Can you work these out from the model? Positions are in its coordinate system, mm. Face numbers are marked on the shaded views. A direction names the side the tool comes from. Coordinates: 2 decimals unless noted, no trailing zeros. Order: outer loops, then holes, each group sorted by start corner. A loop starts at its lowest first (then second) coordinate and runs counter-clockwise, first axis right, second up. Notation, with made-up numbers: (23.25, 83) -> (48.25, 83) arc R12 cw to (48.25, 94) -> close; hole circle Ø5 at (-6, 81.5). An arc over 180 degrees is marked (long way). Write item = value, one per line.
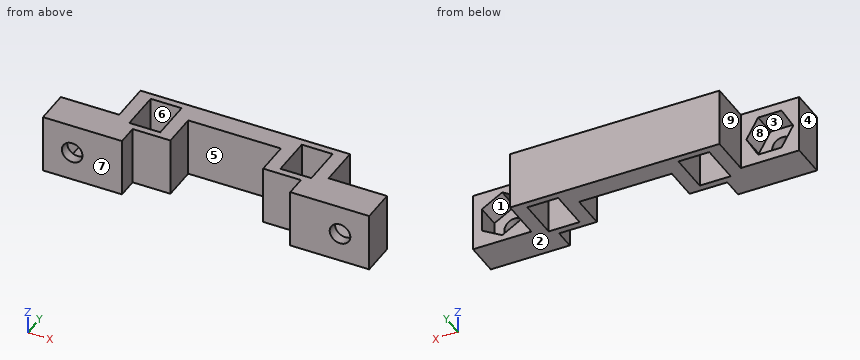
```python
from build123d import *

# Parameters (mm, degrees)
SKETCH1_W           = 8.5
SKETCH1_H           = 8.5
BOSS_EXTRUDE1_DEPTH = 3.5
SKETCH2_W           = 8.5
SKETCH2_H           = 8.5
SKETCH2_R           = 1.5
BOSS_EXTRUDE2_DEPTH = 1.5
SKETCH3_W           = 8.5
SKETCH3_H           = 5
BOSS_EXTRUDE3_DEPTH = 3
SKETCH4_W           = 3
SKETCH4_H           = 8.5
BOSS_EXTRUDE4_DEPTH = 6
SKETCH5_W           = 8.5
SKETCH5_H           = 3
BOSS_EXTRUDE5_DEPTH = 27.5
SKETCH6_W           = 3
SKETCH6_H           = 8.5
BOSS_EXTRUDE6_DEPTH = 8
SKETCH7_W           = 8.5
SKETCH7_H           = 5
BOSS_EXTRUDE7_DEPTH = 8.5
CUT_EXTRUDE1_DEPTH  = 3.5
SKETCH10_R          = 1.5
CUT_EXTRUDE3_DEPTH  = 3.5
BOSS_EXTRUDE8_REACH = 38
SKETCH15_W          = 8.5
SKETCH15_H          = 5
SKETCH16_W          = 4.5
SKETCH16_H          = 6
CUT_EXTRUDE4_DEPTH  = 10
SKETCH17_W          = 13.5
SKETCH17_H          = 5
CUT_EXTRUDE5_DEPTH  = 10


with BuildPart() as part:
    # Sketch1 → Boss-Extrude1 (new body)
    with BuildSketch(Plane(origin=(0, 0, 0), x_dir=(1, 0, 0), z_dir=(0, 1, 0))):
        with Locations((4.25, 4.25)):
            Rectangle(SKETCH1_W, SKETCH1_H)
        Polygon((5.985496764, 7.195964334), (2.575496764, 7.195964334), (0.870496764, 4.242817707), (2.575496764, 1.28967108), (5.985496764, 1.28967108), (7.690496764, 4.242817707), align=None, mode=Mode.SUBTRACT)
    extrude(amount=BOSS_EXTRUDE1_DEPTH)

    # Sketch2 → Boss-Extrude2 (add)
    with BuildSketch(Plane.XZ):
        with Locations((4.25, -4.25)):
            Rectangle(SKETCH2_W, SKETCH2_H)
        with Locations((4.25, -4.25)):
            Circle(SKETCH2_R, mode=Mode.SUBTRACT)
    extrude(amount=BOSS_EXTRUDE2_DEPTH)

    # Sketch3 → Boss-Extrude3 (add)
    with BuildSketch(Plane(origin=(8.5, 0, 0), x_dir=(0, 0, -1), z_dir=(1, 0, 0))):
        with Locations((4.25, 1)):
            Rectangle(SKETCH3_W, SKETCH3_H)
    extrude(amount=BOSS_EXTRUDE3_DEPTH)

    # Sketch4 → Boss-Extrude4 (add)
    with BuildSketch(Plane(origin=(0, 3.5, 0), x_dir=(1, 0, 0), z_dir=(0, 1, 0))):
        with Locations((10, 4.25)):
            Rectangle(SKETCH4_W, SKETCH4_H)
    extrude(amount=BOSS_EXTRUDE4_DEPTH)

    # Sketch5 → Boss-Extrude5 (add)
    with BuildSketch(Plane(origin=(11.5, 0, 0), x_dir=(0, 0, -1), z_dir=(1, 0, 0))):
        with Locations((4.25, 8)):
            Rectangle(SKETCH5_W, SKETCH5_H)
    extrude(amount=BOSS_EXTRUDE5_DEPTH)

    # Sketch6 → Boss-Extrude6 (add)
    with BuildSketch(Plane.XZ.offset(-6.5)):
        with Locations((37.5, -4.25)):
            Rectangle(SKETCH6_W, SKETCH6_H)
    extrude(amount=BOSS_EXTRUDE6_DEPTH)

    # Sketch7 → Boss-Extrude7 (add)
    with BuildSketch(Plane(origin=(39, 0, 0), x_dir=(0, 0, -1), z_dir=(1, 0, 0))):
        with Locations((4.25, 1)):
            Rectangle(SKETCH7_W, SKETCH7_H)
    extrude(amount=BOSS_EXTRUDE7_DEPTH)

    # Sketch8 → Cut-Extrude1 (cut)
    with BuildSketch(Plane(origin=(0, 3.5, 0), x_dir=(1, 0, 0), z_dir=(0, 1, 0))):
        Polygon((46.203146627, 5.955), (43.25, 7.66), (40.296853373, 5.955), (40.296853373, 2.545), (43.25, 0.84), (46.203146627, 2.545), align=None)
    extrude(amount=-CUT_EXTRUDE1_DEPTH, mode=Mode.SUBTRACT)

    # Sketch10 → Cut-Extrude3 (cut)
    with BuildSketch(Plane(origin=(0, 0, 0), x_dir=(1, 0, 0), z_dir=(0, 1, 0))):
        with Locations((43.25, 4.25)):
            Circle(SKETCH10_R)
    extrude(amount=-CUT_EXTRUDE3_DEPTH, mode=Mode.SUBTRACT)

    # Sketch15 → Boss-Extrude8 (add, up to next)
    with BuildSketch(Plane(origin=(11.5, 0, 0), x_dir=(0, 0, -1), z_dir=(1, 0, 0)), mode=Mode.PRIVATE) as boss_extrude8_sk1:
        with Locations((4.25, 4)):
            Rectangle(SKETCH15_W, SKETCH15_H)
    boss_extrude8_tool1 = extrude(boss_extrude8_sk1.sketch, amount=BOSS_EXTRUDE8_REACH, mode=Mode.PRIVATE) - part.part
    add(boss_extrude8_tool1.solids().sort_by_distance((11.5, 4, -4.25))[0])

    # Sketch16 → Cut-Extrude4 (cut)
    with BuildSketch(Plane.XY):
        with Locations((12.75, 5.5)):
            Rectangle(SKETCH16_W, SKETCH16_H)
        with Locations((34.75, 5.5)):
            Rectangle(SKETCH16_W, SKETCH16_H)
    extrude(amount=-CUT_EXTRUDE4_DEPTH, mode=Mode.SUBTRACT)

    # Sketch17 → Cut-Extrude5 (cut)
    with BuildSketch(Plane.XY):
        with Locations((23.75, 4)):
            Rectangle(SKETCH17_W, SKETCH17_H)
    extrude(amount=-CUT_EXTRUDE5_DEPTH, mode=Mode.SUBTRACT)


solid = part.part
```
Item 1: If we mould it in two halves opening along Z, with no side actions, what happens to the marked faces 1, 2, 3 and 4? For each: pulls with the +Z half, pulls with the -Z half, needs draft (parallel to the pull), parting line crosses it, or undercut.
A:
face_1 = undercut
face_2 = pulls with the -Z half
face_3 = undercut
face_4 = needs draft
Item 2: I want a section at B-B, the plane y = 4. Please give me the cut outline in (x, z), plus the area to 3 significant figures.
A:
outline = (8.5, -8.5) -> (10.5, -8.5) -> (10.5, 0) -> (8.5, 0) -> close; (15, -8.5) -> (17, -8.5) -> (17, 0) -> (15, 0) -> close; (30.5, -8.5) -> (32.5, -8.5) -> (32.5, 0) -> (30.5, 0) -> close; (37, -8.5) -> (39, -8.5) -> (39, 0) -> (37, 0) -> close
area = 68.0 mm2
Item 3: I want a section at A-A, the plane x = 4.25. Please give me the cut outline in (y, z), plus the area to 3 significant figures.
A:
outline = (-1.5, -8.5) -> (3.5, -8.5) -> (3.5, -7.2) -> (0, -7.2) -> (0, -5.75) -> (-1.5, -5.75) -> close; (-1.5, -2.75) -> (0, -2.75) -> (0, -1.29) -> (3.5, -1.29) -> (3.5, 0) -> (-1.5, 0) -> close
area = 17.3 mm2
Item 4: If I drill on probe 1 along X at (y, z) = (7.5, -0.5); probe 2 along X at (y, z) = (4.5, -0.5); probe 3 along Z at (x, y) = (43.25, -1), over which ranges is the centre line in solid material (lowest first)?
A:
probe_1 = 8.5 to 10.5, 15 to 32.5, 37 to 39
probe_2 = 8.5 to 10.5, 15 to 17, 30.5 to 32.5, 37 to 39
probe_3 = -8.5 to -5.75, -2.75 to 0
Item 5: I want a section at C-C, the plane z = -1.75. Give the number of separate pieces and of enclosed holes in the cut face, plus the area to 3 significant figures.
A:
separate_pieces = 1
enclosed_holes = 2
area = 201 mm2
Item 6: I'm going to push flat-ended pins straight in: P1, Ø3, axis at y = 7.5, z = -3.5, coming from the -X side; P2, Ø2.5, axis at x = 4, y = 1.5, coming from the +Z side; P3, Ø1, axis at x = 22, z = -7, coming from the -Y side. Where does each tip first touch, or does it pass through?
A:
P1 = 8.5
P2 = 0
P3 = 6.5
Item 7: For the marked faces 5, 6, 7, 8 and 9, which set-ups out of +Z, -Z, +X, -X, +Y, -Y let a thin tool reach every point of the face, with its end or its side?
A:
face_5 = +Z, -Z, -Y
face_6 = +Z, -Z
face_7 = +Z, -Z, +X, -X, -Y
face_8 = +Y
face_9 = +Z, -Z, -X, +Y
